```python
from build123d import *

# Parameters (mm, degrees)
ESBO_O1_R                = 0.85
RESSALTO_EXTRUS_O1_DEPTH = 8
CHANFRO1_SIZE            = 0.5
CHANFRO1_SIZE2           = 0.832139741
ESBO_O2_R                = 2.5
RESSALTO_EXTRUS_O2_DEPTH = 0.4
ESBO_O3_R                = 2.1
RESSALTO_EXTRUS_O3_DEPTH = 1
FILETE1_R                = 0.5
CORTE_EXTRUS_O1_DEPTH    = 1


with BuildPart() as part:
    # Esboço1 → Ressalto-extrusão1 (new body)
    with BuildSketch(Plane.XY):
        Circle(ESBO_O1_R)
    extrude(amount=RESSALTO_EXTRUS_O1_DEPTH)

    # Chanfro1
    chanfro1_edges = [part.edges().sort_by_distance(p)[0] for p in [
        (-0.85, 0, 8),
    ]]
    chanfro1_side = [part.faces().sort_by_distance(p)[0] for p in [
        (-0.85, 0, 4),
    ]]
    chamfer(chanfro1_edges, length=CHANFRO1_SIZE, length2=CHANFRO1_SIZE2, reference=chanfro1_side[0])

    # Esboço2 → Ressalto-extrusão2 (add)
    with BuildSketch(Plane(origin=(0, 0, 0), x_dir=(-1, 0, 0), z_dir=(0, 0, -1))):
        Circle(ESBO_O2_R)
    extrude(amount=RESSALTO_EXTRUS_O2_DEPTH)

    # Esboço3 → Ressalto-extrusão3 (add)
    with BuildSketch(Plane(origin=(0, 0, -0.4), x_dir=(-1, 0, 0), z_dir=(0, 0, -1))):
        Circle(ESBO_O3_R)
    extrude(amount=RESSALTO_EXTRUS_O3_DEPTH)

    # Filete1
    filete1_edges = [part.edges().sort_by_distance(p)[0] for p in [
        (2.1, 0, -1.4),
    ]]
    fillet(filete1_edges, radius=FILETE1_R)

    # Esboço4 → Corte-extrusão1 (cut)
    with BuildSketch(Plane(origin=(0, 0, -1.4), x_dir=(-1, 0, 0), z_dir=(0, 0, -1))):
        with BuildLine():
            Line((-0.6, 0.3), (-1.15, 0.3))
            Line((-1.15, 0.3), (-1.15, -0.3))
            Line((-1.15, -0.3), (-0.6, -0.3))
            ThreePointArc((-0.6, -0.3), (-0.387867966, -0.387867966), (-0.3, -0.6))
            Line((-0.3, -0.6), (-0.3, -1.15))
            Line((-0.3, -1.15), (0.3, -1.15))
            Line((0.3, -1.15), (0.3, -0.6))
            ThreePointArc((0.3, -0.6), (0.387867966, -0.387867966), (0.6, -0.3))
            Line((0.6, -0.3), (1.15, -0.3))
            Line((1.15, -0.3), (1.15, 0.3))
            Line((1.15, 0.3), (0.6, 0.3))
            ThreePointArc((0.6, 0.3), (0.387867966, 0.387867966), (0.3, 0.6))
            Line((0.3, 0.6), (0.3, 1.15))
            Line((0.3, 1.15), (-0.3, 1.15))
            Line((-0.3, 1.15), (-0.3, 0.6))
            ThreePointArc((-0.3, 0.6), (-0.387867966, 0.387867966), (-0.6, 0.3))
        make_face()
    extrude(amount=-CORTE_EXTRUS_O1_DEPTH, mode=Mode.SUBTRACT)


solid = part.part
```
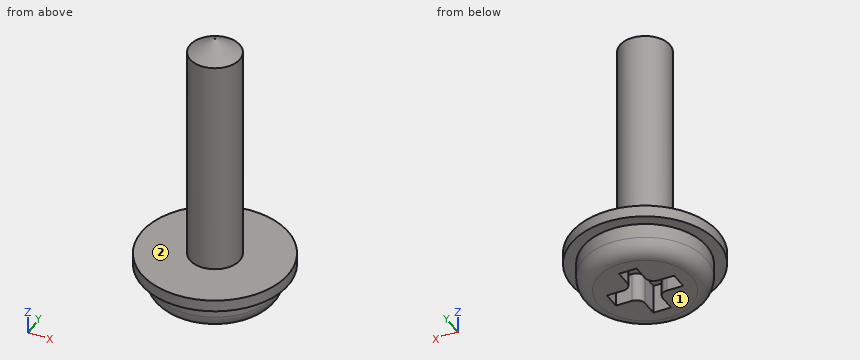
For this review, take the finished solid that the model builds, in its own axes (mm). Face numbers are marked on the shaded views. A direction names the side the tool comes from. Round coordinates to 2 decimals unless told otherwise and drop trailing zeros. Order: outer loops, then holes, each group sorted by start corner. A loop starts at its lowest first (then second) coordinate and runs counter-clockwise, first axis right, second up. Notation, with made-up numbers: (-3, 43.5) -> (55, 43.5) arc R27 cw to (55, 71.5) -> close; hole circle Ø2 at (-26, 45). An arc over 180 degrees is marked (long way). Use a Markdown table: item, result.
Item 1: For pin 1 (3 mm diameter, centred on x = 2, z = 2, fed in from +Y); pin 2 (0.6 mm diameter, centred on x = -1, z = -1, fed in from -Y); pin 3 (0.7 mm diameter, centred on x = 0, z = -1, fed in from +Y), all flat-tipped, find the tip position at first contact; note any pin that passes through.
Resolved:
| item | result |
|---|---|
| pin 1 | stops at y = 0.69 |
| pin 2 | stops at y = -1.98 |
| pin 3 | stops at y = 2.1 |
Item 2: Machinability: for the marked faces 1 and 2, which of the approach directions +Z, -Z, +X, -X, +Y, -Y give a long, thin tool a straight path to every point of the face, cutting with its end or side? Answer none if there is none.
Resolved:
| item | result |
|---|---|
| face 1 | -Z, +X, -X, +Y, -Y |
| face 2 | +Z |
Item 3: For line 1 along Z through (x, y) = (1.5, 0.35); line 2 along X through (y, z) = (-1.1, -0.5); line 3 along Z through (x, y) = (-1.55, 1.65), list the stretches that pass through material, from the lowest coordinate up. Write a range as [from, to].
Resolved:
| item | result |
|---|---|
| line 1 | z = [-1.4, 0] |
| line 2 | x = [-1.79, -0.3], [0.3, 1.79] |
| line 3 | z = [-0.4, 0] |
Item 4: Take a section at A-A (z = 4.5). State the section outline as (x, y) points, plus the area to 3 significant figures.
Resolved:
| item | result |
|---|---|
| outline | circle Ø1.7 at (0, 0) |
| area | 2.27 mm² |
